Geometry check sheet. Reference: drawing and pictorial views, mm from the part's lowest x, y, z. A direction names the side the tool comes from. Coordinates: 2 decimals unless noted, no trailing zeros. Loops run counter-clockwise (first coordinate to the right, second up) from the corner with the lowest first, then second, coordinate; pieces in that order, holes last. Notation, with made-up numbers: (23, 49) -> (60, 49) arc R26 cw to (60, 80) -> close; hole circle Ø11 at (26, 71.5). An arc over 180 degrees is marked (long way). Answer as a JSON object with one key per item and string values.
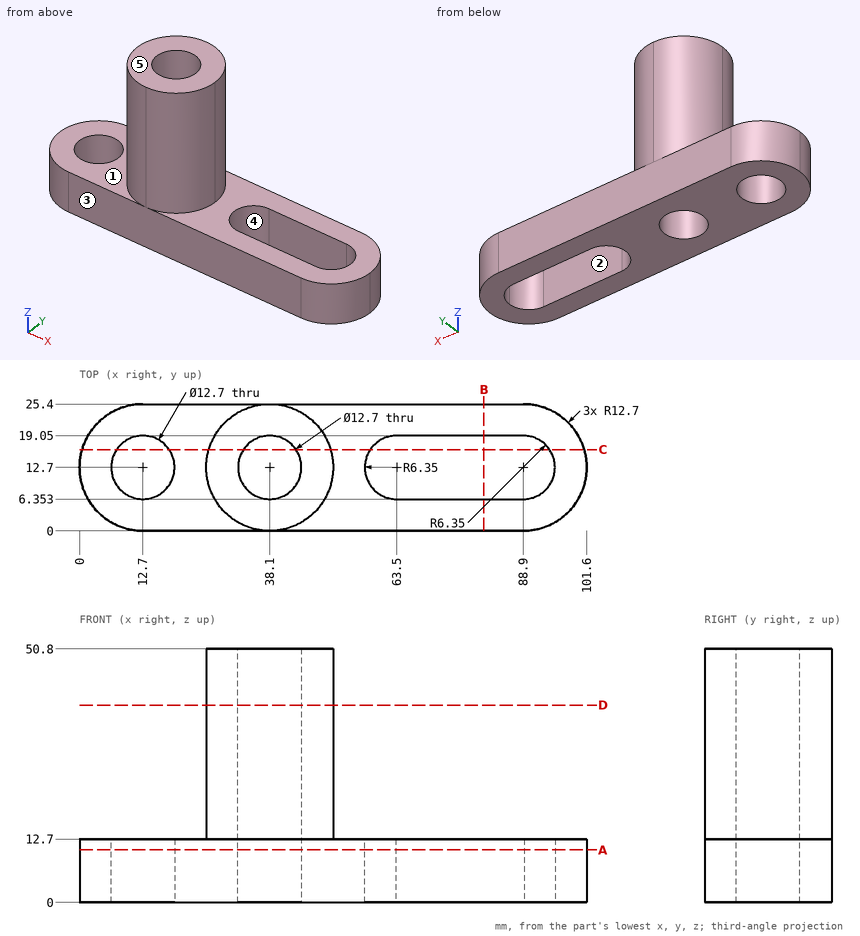
1. Tool access check on the marked faces 4 and 5. Record the directions out of +Z, -Z, +X, -X, +Y, -Y that give a thin tool (end or side, any length) a straight path to the whole face; none if there is none.
Evaluation:
{"face 4": "+Z, -Z", "face 5": "+Z, +X, -X, +Y, -Y"}
2. Section check D-D, the plane z = 39.5. Record the boundary of the cut face in (x, y), then the cut area to 3 significant figures.
Evaluation:
{"outline": "circle Ø25.4 at (38.1, 12.7); hole circle Ø12.7 at (38.1, 12.7)", "area": "380 mm^2"}
3. Mould release check, pull along Y, two halves, no side actions. Record for the marked faces 1, 2 and 3: released by +Y, released by -Y, zero draft, split by the parting line, or undercut.
Evaluation:
{"face 1": "zero draft", "face 2": "undercut", "face 3": "released by -Y"}
4. Section check A-A, the plane z = 10.5. Record the boundary of the cut face in (x, y), then the cut area to 3 significant figures.
Evaluation:
{"outline": "(12.7, 0) -> (88.9, 0) arc R12.7 ccw to (88.9, 25.4) -> (12.7, 25.4) arc R12.7 ccw to start; hole circle Ø12.7 at (12.7, 12.7); hole circle Ø12.7 at (38.1, 12.7); hole (63.31, 6.35) -> (89.09, 6.35) arc R6.35 ccw to (88.9, 19.05) -> (63.5, 19.05) arc R6.35 ccw to start", "area": "1,740 mm^2"}
5. Depth check by flat-ended pin: P1, Ø2, axis at y = 17.5, z = 44, coming from the +X side; P2, Ø1.5, axis at y = 18.5, z = 32, coming from the +X side; P3, Ø12.5, axis at x = 80, y = 13.5, coming from the +Z side. Enter the tip coordinate at first touch or a pass-through.
Evaluation:
{"P1": "stops at x = 50.22", "P2": "stops at x = 49.75", "P3": "stops at z = 12.7"}
6. Section check B-B, the plane x = 81. Record the boundary of the cut face in (y, z).
Evaluation:
{"outline": "(0, 0) -> (6.35, 0) -> (6.35, 12.7) -> (0, 12.7) -> close; (19.05, 0) -> (25.4, 0) -> (25.4, 12.7) -> (19.05, 12.7) -> close"}
7. Section check C-C, the plane y = 16.25. Record the boundary of the cut face in (x, z) (1 decimal), then the cut area to 3 significant figures.
Evaluation:
{"outline": "(0.5, 0) -> (7.4, 0) -> (7.4, 12.7) -> (0.5, 12.7) -> close; (18, 0) -> (32.8, 0) -> (32.8, 50.8) -> (25.9, 50.8) -> (25.9, 12.7) -> (18, 12.7) -> close; (43.4, 0) -> (58.2, 0) -> (58.2, 12.7) -> (50.3, 12.7) -> (50.3, 50.8) -> (43.4, 50.8) -> close; (94.2, 0) -> (101.1, 0) -> (101.1, 12.7) -> (94.2, 12.7) -> close", "area": "1,080 mm^2"}
8. Thickness scan on probe 1 along Y at (x, z) = (12.7, 9.5); probe 2 along X at (y, z) = (18, 7); probe 3 along Z at (x, y) = (57, 2.5). Record the ranges inside material, lowest first. Write a range as from..to.
Evaluation:
{"probe 1": "y = 0..6.35, 19.05..25.4", "probe 2": "x = 1.16..9.2, 16.2..34.6, 41.6..60, 92.4..100.44", "probe 3": "z = 0..12.7"}
